Design review of the part built by this model. Coordinates are the model's own, in mm. A direction names the side the tool comes from. Give positions to 0.01 mm unless a question says otherwise; leave off trailing zeros. Loops run counter-clockwise (first coordinate to the right, second up) from the corner with the lowest first, then second, coordinate; pieces in that order, holes last.
from build123d import *

# Parameters (mm, degrees)
F0_R     = 2.225
F0_R_2   = 1.5
F1_DEPTH = 1.5


# Not quite as in the source:
# - ends of sketch curves that miss each other by under 0.0002 mm in the source are joined


with BuildPart() as f1:
    # F0 (on Top) → F1 (new body)
    with BuildSketch(Plane.XY):
        with BuildLine():
            ThreePointArc((15.5, -50.25), (17.9748737342, -49.2248737342), (19, -46.75))
            Line((19, -46.75), (19, -12.25))
            ThreePointArc((19, -12.25), (18.7803300859, -11.7196699141), (18.25, -11.5))
            ThreePointArc((18.25, -11.5), (17.7196699141, -11.2803300859), (17.5, -10.75))
            Line((17.5, -10.75), (17.5, 10.75))
            ThreePointArc((17.5, 10.75), (17.7196699141, 11.2803300859), (18.25, 11.5))
            ThreePointArc((18.25, 11.5), (18.7803300859, 11.7196699141), (19, 12.25))
            Line((19, 12.25), (19, 46.75))
            ThreePointArc((19, 46.75), (17.9748737342, 49.2248737342), (15.5, 50.25))
            Line((15.5, 50.25), (15.167259, 50.25))
            ThreePointArc((15.167259, 50.25), (0, 47.25), (-15.1672590116, 50.2499999718))
            Line((-15.1672590116, 50.2499999718), (-15.5, 50.25))
            ThreePointArc((-15.5, 50.25), (-17.9748737342, 49.2248737342), (-19, 46.75))
            Line((-19, 46.75), (-19, 12.25))
            ThreePointArc((-19, 12.25), (-18.7803300859, 11.7196699141), (-18.25, 11.5))
            ThreePointArc((-18.25, 11.5), (-17.7196699141, 11.2803300859), (-17.5, 10.75))
            Line((-17.5, 10.75), (-17.5, -10.75))
            ThreePointArc((-17.5, -10.75), (-17.7196699141, -11.2803300859), (-18.25, -11.5))
            ThreePointArc((-18.25, -11.5), (-18.7803300859, -11.7196699141), (-19, -12.25))
            Line((-19, -12.25), (-19, -46.75))
            ThreePointArc((-19, -46.75), (-17.9748737342, -49.2248737342), (-15.5, -50.25))
            Line((-15.5, -50.25), (-15.167259, -50.25))
            ThreePointArc((-15.167259, -50.25), (0, -47.249999), (15.1672593636, -50.2499991168))
            Line((15.1672593636, -50.2499991168), (15.5, -50.25))
        make_face()
        with Locations((-9, -41.75)):
            Circle(F0_R, mode=Mode.SUBTRACT)
        with Locations((-15.25, -15.25)):
            Circle(F0_R_2, mode=Mode.SUBTRACT)
        with Locations((9, -41.75)):
            Circle(F0_R, mode=Mode.SUBTRACT)
        with BuildLine():
            Line((-9, -20.25), (9, -20.25))
            Line((9, -20.25), (9, -28.25))
            ThreePointArc((9, -28.25), (0, -37.25), (-9, -28.25))
            Line((-9, -28.25), (-9, -20.25))
        make_face(mode=Mode.SUBTRACT)
        with Locations((15.25, -15.25)):
            Circle(F0_R_2, mode=Mode.SUBTRACT)
        with Locations((-15.25, 15.25)):
            Circle(F0_R_2, mode=Mode.SUBTRACT)
        with Locations((-9, 41.75)):
            Circle(F0_R, mode=Mode.SUBTRACT)
        with Locations((15.25, 15.25)):
            Circle(F0_R_2, mode=Mode.SUBTRACT)
        with BuildLine():
            ThreePointArc((9, 23.25), (8.1213203436, 21.1286796564), (6, 20.25))
            Line((6, 20.25), (-6, 20.25))
            ThreePointArc((-6, 20.25), (-8.1213203436, 21.1286796564), (-9, 23.25))
            Line((-9, 23.25), (-9, 28.25))
            ThreePointArc((-9, 28.25), (0, 37.25), (9, 28.25))
            Line((9, 28.25), (9, 23.25))
        make_face(mode=Mode.SUBTRACT)
        with Locations((9, 41.75)):
            Circle(F0_R, mode=Mode.SUBTRACT)
    extrude(amount=F1_DEPTH)


solid = f1.part
Q1. Take a section at D-D (z = 0.35). Give the number of separate pieces and of enclosed holes in the cut face, plus the area to 3 significant figures.
Results:
separate pieces: 1
enclosed holes: 10
area: 2,990 mm2
Q2. Tool access review of faces 4 (the face through (0.198, -37.248, 0.74)), 5 (the face through (-17.9, 49.3, 0.7)): name each direction out of +Z, -Z, +X, -X, +Y, -Y from which nothing blocks a thin tool from reaching the whole face with its end or side.
Results:
face 4: +Z, -Z
face 5: +Z, -Z, -X, +Y
Q3. Take a section at C-C (y = -27). Give the boundary of the cut face in (x, z).
Results:
outline: (-19, 0) - (-9, 0) - (-9, 1.5) - (-19, 1.5) - close; (9, 0) - (19, 0) - (19, 1.5) - (9, 1.5) - close
Q4. Take a section at B-B (x = 0). Give the boundary of the cut face in (y, z).
Results:
outline: (-47.25, 0) - (-37.25, 0) - (-37.25, 1.5) - (-47.25, 1.5) - close; (-20.25, 0) - (20.25, 0) - (20.25, 1.5) - (-20.25, 1.5) - close; (37.25, 0) - (47.25, 0) - (47.25, 1.5) - (37.25, 1.5) - close
Q5. Take a section at A-A (y = 15.25). Give the boundary of the cut face in (x, z), plus the area to 3 significant figures.
Results:
outline: (-19, 0) - (-16.75, 0) - (-16.75, 1.5) - (-19, 1.5) - close; (-13.75, 0) - (13.75, 0) - (13.75, 1.5) - (-13.75, 1.5) - close; (16.75, 0) - (19, 0) - (19, 1.5) - (16.75, 1.5) - close
area: 48.0 mm2
Q6. Wall thickness on line 1 (Y direction, x = 15.25, z = 1.15); line 2 (Y direction, x = -2.5, z = 0.15); line 3 (Y direction, x = 8, z = 0.95): over which ranges is each line inside the solid? List them lowest first.
Results:
line 1: y = -50.25 to -16.75, -13.75 to 13.75, 16.75 to 50.25
line 2: y = -47.33 to -36.9, -20.25 to 20.25, 36.9 to 47.33
line 3: y = -48.06 to -43.74, -39.76 to -32.37, -20.25 to 21.01, 32.37 to 39.76, 43.74 to 48.06
Q7. Insertion check: pin 1 (2.5 mm diameter, centred on x = -15.25, y = 15.25, fed in from +Z); pin 2 (0.8 mm diameter, centred on x = 4, z = 1, fed in from -Y). Each pin has a flat end and moves straight along its axis. Give the tip position at first contact, or say it passes through.
Results:
pin 1: passes through
pin 2: stops at y = -47.49
Q8. Draft analysis for pull direction X (two halves, no side actions). For faces 1 (the face through (-10.64, 43.254, 0.74)), 2 (the face through (0, 1, 1.5)), 3 (the face through (-18, -49.2, 0.7)), state which applies: pulls with the +X half, pulls with the -X half, needs draft (parallel to the pull), parting line crosses it, or undercut.
Results:
face 1: undercut
face 2: needs draft
face 3: pulls with the -X half
